Geometry check sheet. Reference: drawing and pictorial views, mm from the part's lowest x, y, z. A direction names the side the tool comes from. Coordinates: 2 decimals unless noted, no trailing zeros. Write each loop counter-clockwise with the first axis right and the second up, starting at its lowest first coordinate (ties: lowest second). Pieces come first, ordered by that corner, then holes. Notation, with made-up numbers: (-6.75, 62) -> (25.25, 62) arc R13 cw to (25.25, 71) -> close; hole circle Ø2 at (-7, -0.5). An arc over 180 degrees is marked (long way). Put each result on its own line as item: value.
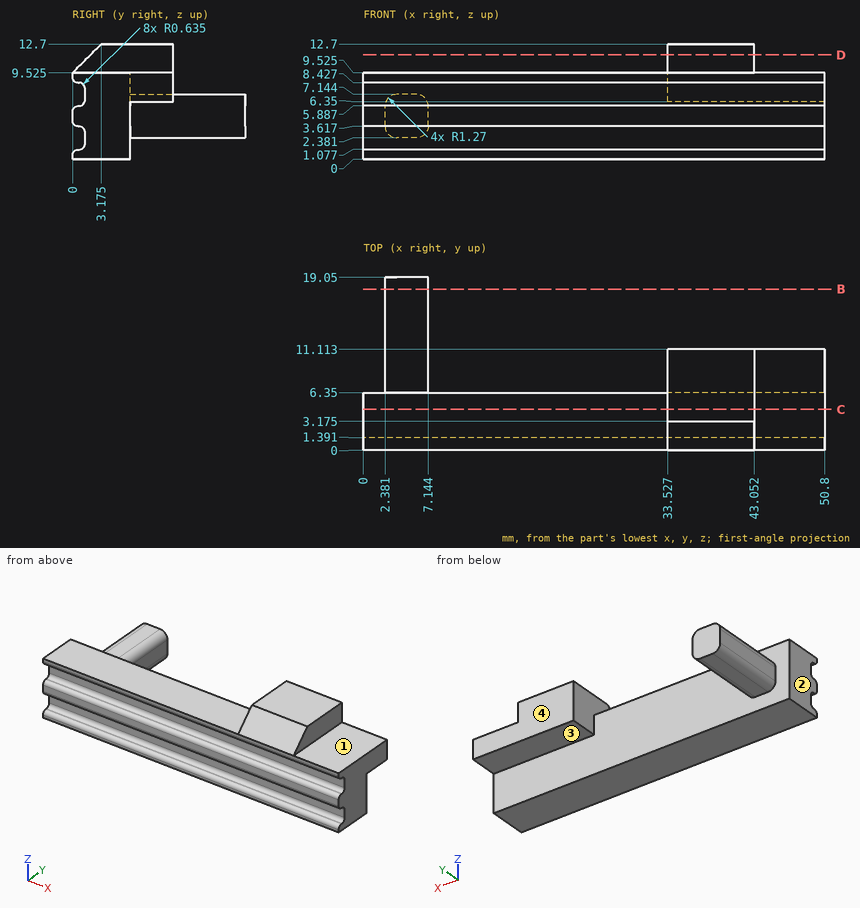
Q1. Material ranges on line 1 along Y through (x, z) = (12.5, 7.75); line 2 along X through (y, z) = (17.75, 5.5); line 3 along Z through (x, y) = (42.5, 6.5), recorded low to high.
Recorded:
line 1: y = 1.39 to 6.35
line 2: x = 2.38 to 7.14
line 3: z = 6.35 to 12.7
Q2. Cross-section at C-C (y = 4.5). Record the cut outline in (x, z) (1 decimal), plus the area to 3 significant figures.
Recorded:
outline: (0, 0) -> (50.8, 0) -> (50.8, 9.5) -> (43.1, 9.5) -> (43.1, 12.7) -> (33.5, 12.7) -> (33.5, 9.5) -> (0, 9.5) -> close
area: 514 mm2
Q3. Cross-section at B-B (y = 17.75). Record the cut outline in (x, z), plus the area to 3 significant figures.
Recorded:
outline: (2.38, 3.65) arc R1.27 ccw to (3.65, 2.38) -> (5.87, 2.38) arc R1.27 ccw to (7.14, 3.65) -> (7.14, 5.87) arc R1.27 ccw to (5.87, 7.14) -> (3.65, 7.14) arc R1.27 ccw to (2.38, 5.87) -> close
area: 21.3 mm2
Q4. Tool access check on the marked faces 1, 2, 3 and 4. Record the directions out of +Z, -Z, +X, -X, +Y, -Y that give a thin tool (end or side, any length) a straight path to the whole face; none if there is none.
Recorded:
face 1: +Z, +X, +Y, -Y
face 2: +Z, -Z, -X, +Y, -Y
face 3: -Z, +X, +Y
face 4: +Z, -Z, +X, +Y
Q5. Depth check by flat-ended pin: P1, Ø1.4, axis at x = 13.5, z = 7.5, coming from the -Y side; P2, Ø1.8, axis at x = 5, y = 12.5, coming from the +Z side; P3, Ø1.1, axis at y = 10.5, z = 4.5, coming from the +X side. Enter the tip coordinate at first touch or a pass-through.
Recorded:
P1: stops at y = 1.24
P2: stops at z = 7.14
P3: stops at x = 7.14
Q6. Cross-section at D-D (z = 11.5). Record the cut outline in (x, y) (1 decimal).
Recorded:
outline: (33.5, 2) -> (43.1, 2) -> (43.1, 11.1) -> (33.5, 11.1) -> close
